```python
from build123d import *

# Parameters (mm, degrees)
SKETCH1_W           = 300
SKETCH1_H           = 150
BOSS_EXTRUDE1_DEPTH = 50
SKETCH2_R           = 25
CUT_EXTRUDE1_DEPTH  = 151


with BuildPart() as part:
    # Sketch1 → Boss-Extrude1 (new body, symmetric)
    with BuildSketch(Plane(origin=(0, 0, 0), x_dir=(1, 0, 0), z_dir=(0, 1, 0))):
        Rectangle(SKETCH1_W, SKETCH1_H)
    extrude(amount=BOSS_EXTRUDE1_DEPTH, both=True)

    # Sketch2 → Cut-Extrude1 (cut, through all)
    with BuildSketch(Plane.XY.offset(75)):
        Circle(SKETCH2_R)
    extrude(amount=-CUT_EXTRUDE1_DEPTH, mode=Mode.SUBTRACT)


solid = part.part
```
Part model, mm, in its own coordinate system. Coordinates: 2 decimals unless noted, no trailing zeros. Write each loop counter-clockwise with the first axis right and the second up, starting at its lowest first coordinate (ties: lowest second). Pieces come first, ordered by that corner, then holes.
Item 1: Slice it at C-C (z = 17.5). Write the cut outline in (x, y), and give its area (3 significant figures).
Item 2: Slice it at A-A (x = 0). Write the cut outline in (y, z), and give its area (3 significant figures).
Item 3: Mould opens along Y. For faces 1 (the face through (-150, 1, 1)), 2 (the face through (-2, 50, -1)), 3 (the face through (23.846, 7.509, 1.05)), 4 (the face through (-2, -50, -1)) say: released by +Y, released by -Y, zero draft, split by the parting line, or undercut.
Item 4: Probe line 1 (Y direction, x = 0, z = -40.5); line 2 (X direction, y = -14.5, z = -67); line 3 (X direction, y = 4, z = 62.5). List the from-to ranges inside material, lowest first.
Item 5: Slice it at B-B (y = 0). Write the cut outline in (x, z), and give its area (3 significant figures).
Results found:
1. outline: (-150, -50) - (150, -50) - (150, 50) - (-150, 50) - close; hole circle Ø50 at (0, 0)
1. area: 28,000 mm2
2. outline: (-50, -75) - (-25, -75) - (-25, 75) - (-50, 75) - close; (25, -75) - (50, -75) - (50, 75) - (25, 75) - close
2. area: 7,500 mm2
3. face 1: zero draft
3. face 2: released by +Y
3. face 3: undercut
3. face 4: released by -Y
4. line 1: y = -50 to -25, 25 to 50
4. line 2: x = -150 to -20.37, 20.37 to 150
4. line 3: x = -150 to -24.68, 24.68 to 150
5. outline: (-150, -75) - (-25, -75) - (-25, 75) - (-150, 75) - close; (25, -75) - (150, -75) - (150, 75) - (25, 75) - close
5. area: 37,500 mm2
